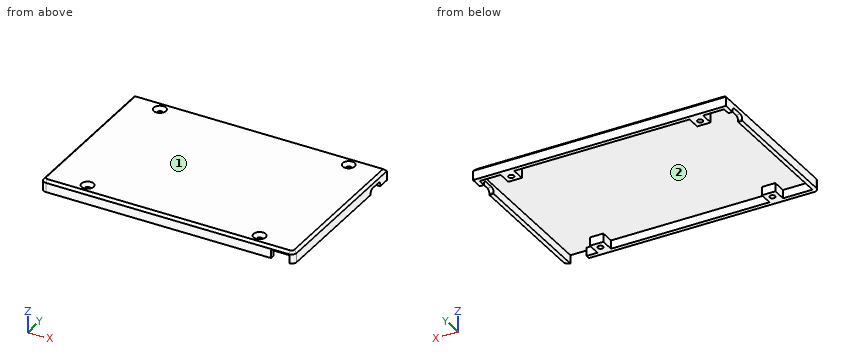
Autodesk Inventor part; units mm, degrees
ref_plane "YZ Plane" through (0, 0, 0) normal (1, 0, 0) x (0, 1, 0)
ref_plane "XZ Plane" through (0, 0, 0) normal (0, 1, 0) x (-1, 0, 0)
ref_plane "XY Plane" through (0, 0, 0) normal (0, 0, 1) x (1, 0, 0)
sketch "Sketch1" plane through (0, 0, 0) normal (0, 0, 1) x (1, 0, 0)
  line L0 (-49.9648, 36.7279) -> (100.0352, 36.7279)
  line L1 (100.0352, 36.7279) -> (100.0352, -60.5221)
  line L2 (100.0352, -60.5221) -> (-49.9648, -60.5221)
  line L3 (-49.9648, -60.5221) -> (-49.9648, 36.7279)
  point P0 (0, 0)
  dimension "d0" = 150
  dimension "d1" = 97.25
extrude "Extrusion1" add sketch "Sketch1" along normal blind 7
sketch "Sketch2" plane through (0, 0, 0) normal (0, 0, -1) x (-1, 0, 0)
  line L0 (47.4648, -58.0221) -> (-97.5352, -58.0221)
  line L1 (-97.5352, -58.0221) -> (-97.5352, 34.2279)
  line L2 (-97.5352, 34.2279) -> (47.4648, 34.2279)
  line L3 (47.4648, 34.2279) -> (47.4648, -58.0221)
  line L4 (49.9648, -60.5221) -> (-100.0352, -60.5221)
  line L5 (-100.0352, -60.5221) -> (-100.0352, 36.7279)
  line L6 (49.9648, 36.7279) -> (49.9648, -60.5221)
  line L7 (-100.0352, 36.7279) -> (49.9648, 36.7279)
  point P0 (0, 0)
  dimension "d4" = 2.5
  dimension "d5" = 2.5
  dimension "d6" = 2.5
  dimension "d7" = 2.5
extrude "Extrusion2" cut sketch "Sketch2" against normal blind 5 contours L0 L1 L2 L3
sketch "Sketch3" plane through (0, 0, 5) normal (0, 0, -1) x (-1, 0, 0)
  line L0 (47.4648, -58.0221) -> (-97.5352, -58.0221)
  line L1 (29.9648, -58.0221) -> (21.9648, -58.0221)
  line L2 (21.9648, -58.0221) -> (21.9648, -50.0221)
  line L3 (21.9648, -50.0221) -> (29.9648, -50.0221)
  line L4 (29.9648, -50.0221) -> (29.9648, -58.0221)
  line L5 (-80.0352, -58.0221) -> (-72.0352, -58.0221)
  line L6 (-72.0352, -58.0221) -> (-72.0352, -50.0221)
  line L7 (-72.0352, -50.0221) -> (-80.0352, -50.0221)
  line L8 (-80.0352, -50.0221) -> (-80.0352, -58.0221)
  line L9 (34.9648, 26.2279) -> (26.9648, 26.2279)
  line L10 (26.9648, 26.2279) -> (26.9648, 34.2279)
  line L11 (26.9648, 34.2279) -> (34.9648, 34.2279)
  line L12 (34.9648, 34.2279) -> (34.9648, 26.2279)
  line L13 (-77.0352, 26.2279) -> (-85.0352, 26.2279)
  line L14 (-85.0352, 26.2279) -> (-85.0352, 34.2279)
  line L15 (-85.0352, 34.2279) -> (-77.0352, 34.2279)
  line L16 (-77.0352, 34.2279) -> (-77.0352, 26.2279)
  line L17 (-100.0352, -60.5221) -> (-100.0352, 36.7279)
  line L18 (49.9648, 36.7279) -> (49.9648, -60.5221)
  line L19 (-100.0352, 36.7279) -> (49.9648, 36.7279)
  point P0 (0, 0)
  dimension "d10" = 8
  dimension "d11" = 8
  dimension "d12" = 8
  dimension "d13" = 20
  dimension "d14" = 20
  dimension "d15" = 8
  dimension "d16" = 8
  dimension "d17" = 8
  dimension "d18" = 8
  dimension "d19" = 15
  dimension "d20" = 15
  dimension "d21" = 10.5
extrude "Extrusion3" add sketch "Sketch3" along normal up to surface (5 mm away)
sketch "Sketch4" plane through (0, 0, 0) normal (0, 0, -1) x (-1, 0, 0)
  circle A0 centre (25.9648, -54.0221) radius 1.6
  circle A1 centre (-76.0352, -54.0221) radius 1.6
  line L0 (49.9648, 36.7279) -> (49.9648, -60.5221)
  line L1 (49.9648, -60.5221) -> (-100.0352, -60.5221)
  line L2 (-100.0352, -60.5221) -> (-100.0352, 36.7279)
  circle A2 centre (30.9648, 30.2279) radius 1.6
  circle A3 centre (-81.0352, 30.2279) radius 1.6
  line L3 (-100.0352, 36.7279) -> (49.9648, 36.7279)
  point P0 (0, 0)
  dimension "d24" = 3.2
  dimension "d25" = 3.2
  dimension "d26" = 24
  dimension "d27" = 6.5
  dimension "d28" = 24
  dimension "d29" = 6.5
  dimension "d30" = 3.2
  dimension "d31" = 3.2
  dimension "d32" = 19
  dimension "d33" = 6.5
  dimension "d34" = 6.5
  dimension "d35" = 19
extrude "Extrusion4" cut sketch "Sketch4" against normal through all contours A0 | A1 | A2 | A3
fillet "Fillet1" radius 3 2 edges at (100.0352, -60.5221, 3.5) (-49.9648, -60.5221, 3.5)
sketch "Sketch5" plane through (100.0352, 36.7279, 7) normal (1, 0, 0) x (0, 0, -1)
  line L0 (7, -17) -> (4, -17)
  line L1 (4, -17) -> (4, -7)
  line L2 (4, -7) -> (7, -7)
  line L3 (7, -7) -> (7, -17)
  line L4 (7, -94.25) -> (7, 0)
  line L5 (7, 0) -> (0, 0)
  point P0 (7, -36.7279)
  dimension "d39" = 3
  dimension "d40" = 7
  dimension "d41" = 10
extrude "Extrusion5" cut sketch "Sketch5" against normal up to surface (2.5 mm away)
fillet "Fillet2" radius 2 2 edges at (98.7852, 29.7279, 3) (98.7852, 19.7279, 3)
sketch "Sketch6" plane through (-49.9648, 36.7279, 0) normal (-1, 0, 0) x (0, 0, 1)
  line L0 (0, -2.5) -> (0, -94.75)
  line L1 (0, -7) -> (3, -7)
  line L2 (3, -7) -> (3, -17)
  line L3 (3, -17) -> (0, -17)
  line L4 (0, -17) -> (0, -7)
  line L5 (0, 0) -> (7, 0)
  point P0 (0, -36.7279)
  point P1 (0, -17)
  dimension "d45" = 3
  dimension "d46" = 10
  dimension "d47" = 7
extrude "Extrusion6" cut sketch "Sketch6" against normal up to surface (2.5 mm away)
fillet "Fillet3" radius 2 2 edges at (-48.7148, 29.7279, 3) (-48.7148, 19.7279, 3)
chamfer "Chamfer1" distance 1.5 angle 45 6 edges at (25.0352, 36.7279, 7) (-49.9648, -10.3971, 7) (-49.0861, -59.6434, 7) (25.0352, -60.5221, 7) (99.1566, -59.6434, 7) (100.0352, -10.3971, 7)
sketch "Sketch7" plane through (-46.9648, -60.5221, 0) normal (0, -1, 0) x (1, 0, 0)
  line L0 (147, 0) -> (-3, 0)
  line L1 (133.5, 0) -> (144.5, 0)
  line L2 (144.5, 0) -> (144.5, 5)
  line L3 (144.5, 5) -> (133.5, 5)
  line L4 (133.5, 5) -> (133.5, 0)
  line L5 (147, 0) -> (147, 5.5)
  point P0 (46.9648, 0)
  dimension "d54" = 5
  dimension "d55" = 11
  dimension "d56" = 2.5
extrude "Extrusion7" cut sketch "Sketch7" against normal up to surface (2.5 mm away)
chamfer "Chamfer2" distance 2 angle 45 4 edges at (-29.3648, 30.2279, 7) (-24.3648, -54.0221, 7) (77.6352, -54.0221, 7) (82.6352, 30.2279, 7)
properties part number "e_box_lid"
Could you check a few things on this model? Use its own coordinates, in mm. Face numbers are marked on the shaded views. Round coordinates to 2 decimals unless told otherwise and drop trailing zeros. Loops run counter-clockwise (first coordinate to the right, second up) from the corner with the lowest first, then second, coordinate; pieces in that order, holes last. Notation, with made-up numbers: (-16.5, 88) -> (15.5, 88) arc R22 ccw to (15.5, 124) -> close; hole circle Ø1 at (47.5, -18.75). An arc over 180 degrees is marked (long way). Use CSV: the item, a comma, the result in double quotes.
(1) Suppose I cut it at C-C on x = 89. Write out the boundary of the cut face in (y, z).
Return value:
outline,"(-60.52, 5) -> (34.23, 5) -> (34.23, 0) -> (36.73, 0) -> (36.73, 5.5) -> (35.23, 7) -> (-59.02, 7) -> (-60.52, 5.5) -> close"
(2) If we mould it in two halves opening along Y, with no side actions, what happens to the marked faces 1 and 2? For each: +Y half, -Y half, draft (parallel to the pull), parting line (faces both ways), or undercut.
Return value:
face 1,"draft"
face 2,"undercut"
(3) Suppose I cut it at B-B on y = 5. Write out the boundary of the cut face in (x, z), plus the area to 3 significant figures.
Return value:
outline,"(-49.96, 0) -> (-47.46, 0) -> (-47.46, 5) -> (97.54, 5) -> (97.54, 0) -> (100.04, 0) -> (100.04, 5.5) -> (98.54, 7) -> (-48.46, 7) -> (-49.96, 5.5) -> close"
area,"323 mm²"
(4) Will these pins go through, and if not, where does the flat tip stop? pin 1 Ø4 at (y, z) = (-41.5, 6) entering from -X; pin 2 Ø3 at (x, y) = (-49, 24) entering from -Z; pin 3 Ø8 at (x, y) = (43, -2.5) entering from -Z; pin 4 Ø1.2 at (y, z) = (-59.5, 3) entering from +X.
Return value:
pin 1,"stops at x = -49.96"
pin 2,"stops at z = 3"
pin 3,"stops at z = 5"
pin 4,"stops at x = 99.7"
(5) Suppose I cut it at A-A on x = 21.5. Write out the boundary of the cut face in (y, z).
Return value:
outline,"(-60.52, 0) -> (-58.02, 0) -> (-58.02, 5) -> (34.23, 5) -> (34.23, 0) -> (36.73, 0) -> (36.73, 5.5) -> (35.23, 7) -> (-59.02, 7) -> (-60.52, 5.5) -> close"
(6) If I drill on probe 1 along Y at (x, z) = (39.5, 0.75); probe 2 along X at (y, z) = (-42, 3.25); probe 3 along X at (y, z) = (29.5, 4.5), over which ranges is the centre line in solid material (lowest first)? Write a range as [from, to].
Return value:
probe 1,"y = [-60.52, -58.02], [34.23, 36.73]"
probe 2,"x = [-49.96, -47.46], [97.54, 100.04]"
probe 3,"x = [-49.96, -47.46], [-34.96, -32.39], [-29.54, -26.96], [77.04, 79.61], [82.46, 85.04], [97.54, 100.04]"
